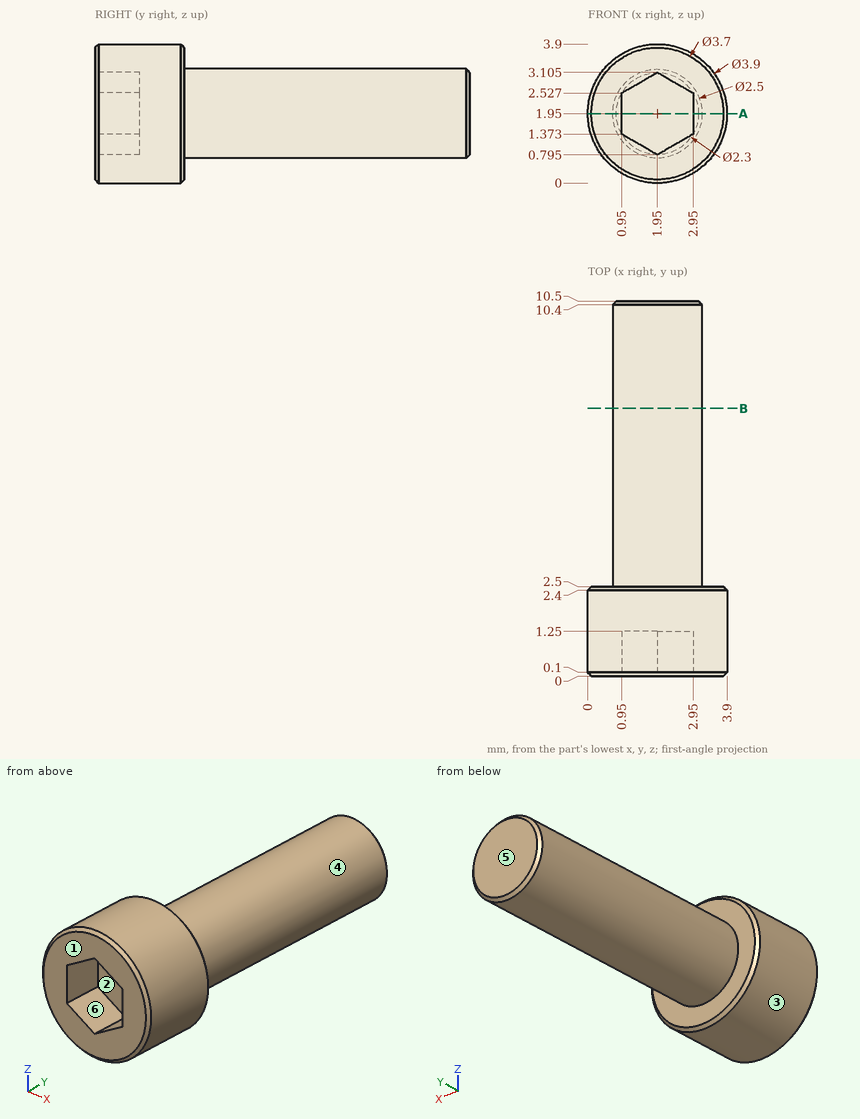
Geometry: see drawing. Coordinates: mm, zero at the bounding-box minimum. A direction names the side the tool comes from. Round coordinates to 2 decimals unless told otherwise and drop trailing zeros. Write each loop counter-clockwise with the first axis right and the second up, starting at its lowest first coordinate (ties: lowest second). Pieces come first, ordered by that corner, then holes.
Item 1: Section query B-B (y = 7.5). Return loops of the section in (x, z).
Item 2: Pin query (flat end, axial travel): P1, Ø2, axis at x = 2.5, y = 4, coming from the +Z side. Return the tip coordinate at first contact, or that it passes through.
Item 3: Material intervals for L1, parallel to Y at x = 0.8, z = 1.05; L2, parallel to Z at x = 2.65, y = 0.5; L3, parallel to X at y = 8, z = 2.8 (1 decimal), sorted ascending.
Item 4: Set-up query: the marked faces 4, 5 and 6. Return all of +Z, -Z, +X, -X, +Y, -Y with unobstructed straight access to the full face (end or side cutting, diameter ignored); none if empty.
Item 5: Mould query, pull axis Z, two halves, no side actions, for the marked faces 1, 2 and 3. Classes: +Z half, -Z half, draft (parallel to the pull), parting line (faces both ways), or undercut.
Item 6: Section query A-A (z = 1.95). Return loops of the section in (x, y).
Completed:
1. outline: circle Ø2.5 at (1.95, 1.95)
2. P1: stops at z = 3.2
3. L1: y = 0 to 2.5
3. L2: z = 0.13 to 1.2, 2.7 to 3.77
3. L3: x = 1 to 2.9
4. face 4: +Y
4. face 5: +Z, -Z, +X, -X, +Y
4. face 6: -Y
5. face 1: draft
5. face 2: undercut
5. face 3: parting line
6. outline: (0, 0.1) - (0.1, 0) - (0.95, 0) - (0.95, 1.25) - (2.95, 1.25) - (2.95, 0) - (3.8, 0) - (3.9, 0.1) - (3.9, 2.4) - (3.8, 2.5) - (3.2, 2.5) - (3.2, 10.4) - (3.1, 10.5) - (0.8, 10.5) - (0.7, 10.4) - (0.7, 2.5) - (0.1, 2.5) - (0, 2.4) - close
